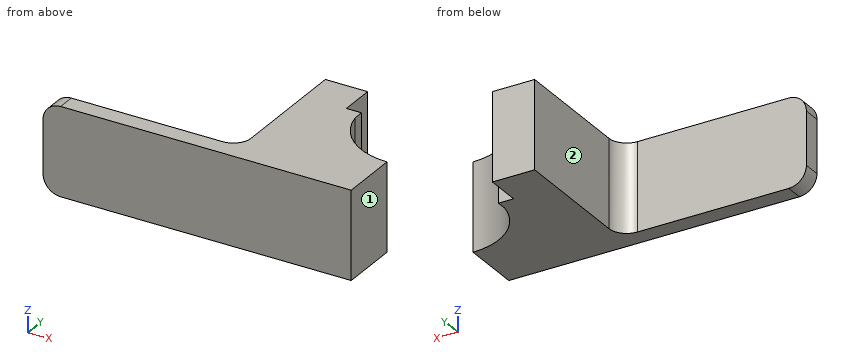
from build123d import *

# Parameters (mm, degrees)
BOSS_EXTRUDE1_DEPTH = 635
FILLET5_R           = 127
FILLET6_R           = 127


with BuildPart() as part:
    # Sketch3 → Boss-Extrude1 (new body)
    with BuildSketch(Plane.XY):
        with BuildLine():
            Line((-2079.212661728, -769.863228), (-860.012661728, -769.863228))
            ThreePointArc((-860.012661728, -769.863228), (-770.210100518, -732.665789211), (-733.012661728, -642.863228))
            Line((-733.012661728, -642.863228), (-733.012661728, 246.136772))
            Line((-733.012661728, 246.136772), (-428.150553924, 246.136772))
            Line((-428.150553924, 246.136772), (-428.150553924, -7.863228))
            Line((-428.150553924, -7.863228), (-326.612661728, -7.863228))
            Line((-326.612661728, -7.863228), (-318.929679791, -7.863228))
            Line((-318.929679791, -7.863228), (-318.929679791, -84.063228))
            ThreePointArc((-318.929679791, -84.063228), (-157.578570713, -360.389072068), (143.287338272, -469.33794683))
            Line((143.287338272, -469.33794683), (143.287338272, -896.863228))
            Line((143.287338272, -896.863228), (-2079.212661728, -896.863228))
            Line((-2079.212661728, -896.863228), (-2079.212661728, -769.863228))
        make_face()
    extrude(amount=BOSS_EXTRUDE1_DEPTH)

    # Fillet5
    fillet5_edges = [part.edges().sort_by_distance(p)[0] for p in [
        (-2079.212661728, -833.363228, 635),
    ]]
    fillet(fillet5_edges, radius=FILLET5_R)

    # Fillet6
    fillet6_edges = [part.edges().sort_by_distance(p)[0] for p in [
        (-2079.212661728, -833.363228, 0),
    ]]
    fillet(fillet6_edges, radius=FILLET6_R)


solid = part.part
The model under review builds one solid part; all positions refer to its coordinate system, in mm. Face numbers are marked on the shaded views. A direction names the side the tool comes from. Give positions to 0.01 mm unless a question says otherwise; leave off trailing zeros. Loops run counter-clockwise (first coordinate to the right, second up) from the corner with the lowest first, then second, coordinate; pieces in that order, holes last. Notation, with made-up numbers: (-24, -24) -> (17, -24) arc R22 cw to (17, -18) -> close; hole circle Ø9 at (-34, 11.5). An arc over 180 degrees is marked (long way). Write each question's results on one line, items separated by ' | '.
1) For line 1 along X through (y, z) = (48, 74.5); line 2 along X through (y, z) = (-57.5, 201.5); line 3 along Y through (x, z) = (-908.5, 126.5), list the stretches that pass through material, from the lowest coordinate up. Write a range as from..to.
Conclusion:
line 1: x = -733.01..-428.15 | line 2: x = -733.01..-318.93 | line 3: y = -896.86..-769.86
2) Insertion check: pin 1 Ø6 at (y, z) = (37.5, 488) entering from -X; pin 2 Ø1 at (x, z) = (-783.5, 150) entering from +Y; pin 3 Ø6 at (y, z) = (30, 303.5) entering from +X. Each pin has a flat end and moves straight along its axis. Give the tip position at first contact, or say it passes through.
Conclusion:
pin 1: stops at x = -733.01 | pin 2: stops at y = -743.85 | pin 3: stops at x = -428.15
3) Tool access review of the marked faces 1 and 2: name each direction out of +Z, -Z, +X, -X, +Y, -Y from which nothing blocks a thin tool from reaching the whole face with its end or side.
Conclusion:
face 1: +Z, -Z, +X, +Y, -Y | face 2: +Z, -Z, -X, +Y
4) Take a section at C-C, the plane y = -256.5. Give the boundary of the cut face in (x, z), plus the area to 3 significant figures.
Conclusion:
outline: (-733.01, 0) -> (-250.06, 0) -> (-250.06, 635) -> (-733.01, 635) -> close | area: 307,000 mm^2
5) Take a section at A-A, the plane x = -385. Give the boundary of the cut face in (y, z), plus the area to 3 significant figures.
Conclusion:
outline: (-896.86, 0) -> (-7.86, 0) -> (-7.86, 635) -> (-896.86, 635) -> close | area: 565,000 mm^2
6) Take a section at B-B, the plane z = 553. Give the boundary of the cut face in (x, y), plus the area to 3 significant figures.
Conclusion:
outline: (-2070.97, -896.86) -> (143.29, -896.86) -> (143.29, -469.34) arc R469.9 cw to (-318.93, -84.06) -> (-318.93, -7.86) -> (-428.15, -7.86) -> (-428.15, 246.14) -> (-733.01, 246.14) -> (-733.01, -642.86) arc R127 cw to (-860.01, -769.86) -> (-2070.97, -769.86) -> close | area: 861,000 mm^2
